from build123d import *

# Parameters (mm, degrees)
SKETCH1_R           = 5
BOSS_EXTRUDE1_DEPTH = 25
SKETCH2_R           = 10
BOSS_EXTRUDE2_DEPTH = 5
SKETCH3_R           = 10
BOSS_EXTRUDE3_DEPTH = 5
FILLET1_R           = 2
FILLET2_R           = 2


with BuildPart() as part:
    # Sketch1 → Boss-Extrude1 (new body, symmetric)
    with BuildSketch(Plane.XY):
        Circle(SKETCH1_R)
    extrude(amount=BOSS_EXTRUDE1_DEPTH, both=True)

    # Sketch2 → Boss-Extrude2 (add)
    with BuildSketch(Plane.XY.offset(25)):
        Circle(SKETCH2_R)
    extrude(amount=BOSS_EXTRUDE2_DEPTH)

    # Sketch3 → Boss-Extrude3 (add)
    with BuildSketch(Plane(origin=(0, 0, -25), x_dir=(-1, 0, 0), z_dir=(0, 0, -1))):
        Circle(SKETCH3_R)
    extrude(amount=BOSS_EXTRUDE3_DEPTH)

    # Fillet1
    fillet1_edges = [part.edges().sort_by_distance(p)[0] for p in [
        (-10, 0, 30),
    ]]
    fillet(fillet1_edges, radius=FILLET1_R)

    # Fillet2
    fillet2_edges = [part.edges().sort_by_distance(p)[0] for p in [
        (10, 0, -30),
    ]]
    fillet(fillet2_edges, radius=FILLET2_R)


solid = part.part
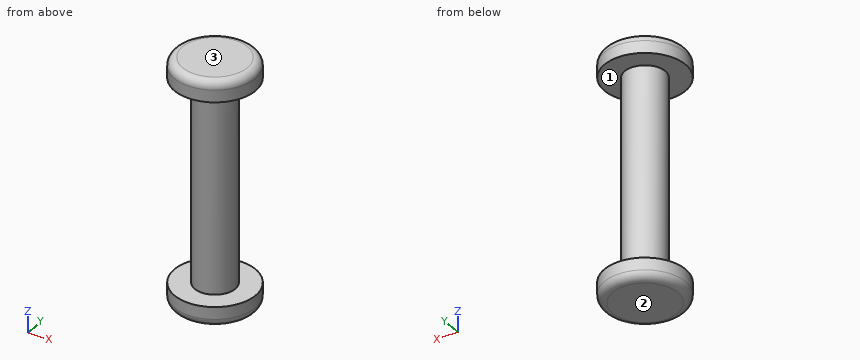
Geometry check sheet. Reference: the model listing, model coordinates, mm. Face numbers are marked on the shaded views. Round coordinates to 2 decimals unless told otherwise and drop trailing zeros. Order: outer loops, then holes, each group sorted by start corner. A loop starts at its lowest first (then second) coordinate and runs counter-clockwise, first axis right, second up. Notation, with made-up numbers: M 89.25,75 L 109.25,75 A17 cw 109.25,95 Z; hole C 2,26 d5. An arc over 180 degrees is marked long. Answer in a Markdown table with one row per item. Add a question column.
Item 1: Material ranges on L1, parallel to Z at x = 6.5, y = -1; L2, parallel to Y at x = 0.25, z = -9.5; L3, parallel to Z at x = 7.25, y = -6, recorded low to high. Write a range as [from, to].
Item 2: Sectioned sample at A-A, the plane y = 0. Enter the section's corners in (x, z), plus the area to 3 significant figures.
Item 3: Depth check by flat-ended pin: pin 1 Ø3 at (x, z) = (-5.5, 20.5) entering from +Y; pin 2 Ø1 at (y, z) = (1, 2.5) entering from +X; pin 3 Ø1.5 at (y, z) = (-2, 19.5) entering from -X. Enter the tip coordinate at first touch or a pass-through.
Item 4: Sectioned sample at C-C, the plane z = -22.5. Enter the section's corners in (x, y).
Item 5: Draft check along Z on the marked faces 1, 2 and 3. Enter one of: released by +Z, released by -Z, zero draft, split by the parting line, or undercut.
Filled in:
| question | item | result |
|---|---|---|
| 1 | L1 | z = [-30, -25], [25, 30] |
| 1 | L2 | y = [-4.99, 4.99] |
| 1 | L3 | z = [-29.42, -25], [25, 29.42] |
| 2 | outline | M -10,-28 A2 ccw -8,-30 L 8,-30 A2 ccw 10,-28 L 10,-25 L 5,-25 L 5,25 L 10,25 L 10,28 A2 ccw 8,30 L -8,30 A2 ccw -10,28 L -10,25 L -5,25 L -5,-25 L -10,-25 Z |
| 2 | area | 697 mm² |
| 3 | pin 1 | stops at y = 3 |
| 3 | pin 2 | stops at x = 4.97 |
| 3 | pin 3 | stops at x = -4.84 |
| 4 | outline | C 0,0 d10 |
| 5 | face 1 | undercut |
| 5 | face 2 | released by -Z |
| 5 | face 3 | released by +Z |
